from build123d import *

# Parameters (mm, degrees)
BOSS_EXTRUDE1_DEPTH            = 13.97
FILLET1_R                      = 1.27
CBORE_FOR_M8_SHCS1_D           = 9
CBORE_FOR_M8_SHCS1_CBORE_D     = 13.5
CBORE_FOR_M8_SHCS1_CBORE_DEPTH = 4
M4_CLEARANCE_HOLE1_D           = 4.3
SKETCH6_R                      = 4.5
CUT_EXTRUDE1_DEPTH             = 4
BOSS_EXTRUDE3_REACH            = 19.794
SKETCH9_R                      = 6.985
SKETCH9_R_2                    = 2.15


with BuildPart() as part:
    # Sketch1 → Boss-Extrude1 (new body)
    with BuildSketch(Plane.XY):
        with BuildLine():
            Line((-8.897, -5), (-8.897, -21.956))
            ThreePointArc((-8.897, -21.956), (-7.755595126, -24.711595126), (-5, -25.853))
            Line((-5, -25.853), (5, -25.853))
            ThreePointArc((5, -25.853), (7.755595126, -24.711595126), (8.897, -21.956))
            Line((8.897, -21.956), (8.897, -5))
            Line((8.897, -5), (8.897, 5))
            ThreePointArc((8.897, 5), (7.755595126, 7.755595126), (5, 8.897))
            Line((5, 8.897), (-5, 8.897))
            ThreePointArc((-5, 8.897), (-7.755595126, 7.755595126), (-8.897, 5))
            Line((-8.897, 5), (-8.897, -5))
        make_face()
    extrude(amount=BOSS_EXTRUDE1_DEPTH)

    # Fillet1
    fillet1_edges = [part.edges().sort_by_distance(p)[0] for p in [
        (-7.755595126, -24.711595126, 13.97),
        (7.755595126, 7.755595126, 0),
        (8.897, -8.478, 0),
        (7.755595126, -24.711595126, 0),
        (0, -25.853, 0),
        (-7.755595126, -24.711595126, 0),
        (-8.897, -8.478, 0),
        (0, -25.853, 13.97),
        (7.755595126, -24.711595126, 13.97),
        (8.897, -8.478, 13.97),
        (7.755595126, 7.755595126, 13.97),
        (0, 8.897, 13.97),
        (-7.755595126, 7.755595126, 13.97),
        (-8.897, -8.478, 13.97),
        (-7.755595126, 7.755595126, 0),
        (0, 8.897, 0),
    ]]
    fillet(fillet1_edges, radius=FILLET1_R)

    # CBORE for M8 SHCS1 (through all)
    with Locations(Plane.XY.offset(13.97)):
        with Locations((0, 0)):
            CounterBoreHole(CBORE_FOR_M8_SHCS1_D / 2, CBORE_FOR_M8_SHCS1_CBORE_D / 2, CBORE_FOR_M8_SHCS1_CBORE_DEPTH)

    # M4 Clearance Hole1 (through all)
    with Locations(Plane(origin=(8.897, 0, 0), x_dir=(0, 0, -1), z_dir=(1, 0, 0))):
        with Locations((-6.985, -18.233)):
            Hole(M4_CLEARANCE_HOLE1_D / 2)

    # Sketch6 → Cut-Extrude1 (cut)
    with BuildSketch(Plane.XY):
        Circle(SKETCH6_R)
        Polygon((-3.75277675, 6.5), (-7.505553499, 0), (-3.75277675, -6.5), (3.75277675, -6.5), (7.505553499, 0), (3.75277675, 6.5), align=None)
        Polygon((-3.25, 5.629165125), (-6.5, 3.75277675), (-6.5, 0), (-6.5, -3.75277675), (-3.25, -5.629165125), (0, -7.505553499), (3.25, -5.629165125), (6.5, -3.75277675), (6.5, 0), (6.5, 3.75277675), (3.25, 5.629165125), (0, 7.505553499), align=None)
        Polygon((6.5, 3.75277675), (4.758330249, 4.758330249), (6.5, 1.741669751), align=None)
        Polygon((6.5, -3.75277675), (6.5, -1.741669751), (4.758330249, -4.758330249), align=None)
        Polygon((3.75277675, -6.5), (4.758330249, -4.758330249), (3.25, -5.629165125), (1.741669751, -6.5), align=None)
        Polygon((1.741669751, 6.5), (3.25, 5.629165125), (4.758330249, 4.758330249), (3.75277675, 6.5), align=None)
        Polygon((-6.5, 1.741669751), (-4.758330249, 4.758330249), (-6.5, 3.75277675), align=None)
        Polygon((-4.758330249, -4.758330249), (-6.5, -1.741669751), (-6.5, -3.75277675), align=None)
        Polygon((-3.25, -5.629165125), (-4.758330249, -4.758330249), (-3.75277675, -6.5), (-1.741669751, -6.5), align=None)
        Polygon((0, -7.505553499), (1.741669751, -6.5), (-1.741669751, -6.5), align=None)
        Polygon((-3.25, 5.629165125), (-1.741669751, 6.5), (-3.75277675, 6.5), (-4.758330249, 4.758330249), align=None)
        Polygon((7.505553499, 0), (6.5, 1.741669751), (6.5, 0), (6.5, -1.741669751), align=None)
        Polygon((-1.741669751, 6.5), (1.741669751, 6.5), (0, 7.505553499), align=None)
        Polygon((-6.5, 0), (-6.5, 1.741669751), (-7.505553499, 0), (-6.5, -1.741669751), align=None)
    extrude(amount=CUT_EXTRUDE1_DEPTH, mode=Mode.SUBTRACT)

    # Sketch9 → Boss-Extrude3 (add, up to next)
    with BuildSketch(Plane.ZY.offset(8.897), mode=Mode.PRIVATE) as boss_extrude3_sk1:
        with Locations((6.985, -18.233)):
            Circle(SKETCH9_R)
        with Locations((6.985, -18.233)):
            Circle(SKETCH9_R_2, mode=Mode.SUBTRACT)
    boss_extrude3_tool1 = extrude(boss_extrude3_sk1.sketch, amount=-BOSS_EXTRUDE3_REACH, mode=Mode.PRIVATE) - part.part
    add(boss_extrude3_tool1.solids().sort_by_distance((-8.897, -18.233, 0.197566))[0])


solid = part.part
The listing builds one solid part. Answer for the finished solid, in the listing's coordinates (mm). A direction names the side the tool comes from. Round coordinates to 2 decimals unless told otherwise and drop trailing zeros. Order: outer loops, then holes, each group sorted by start corner. A loop starts at its lowest first (then second) coordinate and runs counter-clockwise, first axis right, second up. Notation, with made-up numbers: (-28.75, -3.75) - (25.25, -3.75) arc R24 cw to (25.25, 16.25) - close; hole circle Ø9 at (73, 83.25). An arc over 180 degrees is marked (long way). Write item = value, one per line. Start each with the question number.
1) Section C-C, the plane z = 6 is taken. Write down the section's boundary in (x, y).
2) Given pin 1 (4 mm diameter, centred on x = -1, y = 3, fed in from +Z); pin 2 (7.5 mm diameter, centred on x = 3, y = 0, fed in from -Z); pin 3 (8 mm diameter, centred on x = 0, y = 0, fed in from -Z), each flat-ended and moving along its own axis, determine where each tip first touches the part or whether it passes through.
3) Straight lines are drawn through the part: L1, parallel to Y at x = 0, z = 6.05; L2, parallel to Y at x = 1, z = 8; L3, parallel to Y at x = -3.5, z = 1.25. For each, find the intervals that lie inside material, in ascending order.
4) Section A-A, the plane z = 11.5 is taken. Write down the section's boundary in (x, y).
5) Section B-B, the plane y = -17.5 is taken. Write down the section's boundary in (x, z).
6) For faces 1 (the flat face through (4.4, 1.6, 9.97)), 2 (the cylindrical face through (0.59, 4.46, 6.94)), 3 (the flat face through (-6.5, -3, 2)), 4 (the flat face through (0, -25.853, 7)), 5 (the cylindrical face through (-8.126, -20.948, 13.868)), determine the directions among +Z, -Z, +X, -X, +Y, -Y from which every point of the face is accessible in a straight line to the end or side of a thin tool.
7) Section D-D, the plane y = -2.5 is taken. Write down the section's boundary in (x, z).
8) For a pull along X with two mould halves and no side action, classify faces 6 (the cylindrical face through (8.535, -8.289, 0.382)), 7 (the cylindrical face through (0.07, -25.49, 0.38)), 8 (the flat face through (-3, 6.5, 2)) as released by +X, released by -X, zero draft, split by the parting line, or undercut.
Results list:
q1.outline = (-8.9, -25.15) - (-7.24, -25.15) arc R3.9 ccw to (-5, -25.85) - (5, -25.85) arc R3.9 ccw to (8.9, -21.96) - (8.9, -20.14) - (-8.9, -20.14) - close; (-8.9, -16.32) - (8.9, -16.32) - (8.9, 5) arc R3.9 ccw to (5, 8.9) - (-5, 8.9) arc R3.9 ccw to (-8.9, 5) - close; hole circle Ø9 at (0, 0)
q2.pin_1 = 9.97
q2.pin_2 = 4
q2.pin_3 = through
q3.L1 = -25.85 to -20.17, -16.3 to -4.5, 4.5 to 8.9
q3.L2 = -25.85 to -20.13, -16.34 to -4.39, 4.39 to 8.9
q3.L3 = -25.85 to -6.5, 6.5 to 8.9
q4.outline = (-8.9, -23.56) - (-8.55, -23.56) arc R3.9 ccw to (-5, -25.85) - (5, -25.85) arc R3.9 ccw to (8.9, -21.96) - (8.9, 5) arc R3.9 ccw to (5, 8.9) - (-5, 8.9) arc R3.9 ccw to (-8.9, 5) - close; hole circle Ø13.5 at (0, 0)
q5.outline = (-8.9, 0.04) - (-7.94, 0.04) arc R1.27 ccw to (-7.63, 0) - (7.63, 0) arc R1.27 ccw to (8.9, 1.27) - (8.9, 4.96) - (-8.9, 4.96) - close; (-8.9, 9.01) - (8.9, 9.01) - (8.9, 12.7) arc R1.27 ccw to (7.63, 13.97) - (-7.63, 13.97) arc R1.27 ccw to (-7.94, 13.93) - (-8.9, 13.93) - close
q6.face_1 = +Z
q6.face_2 = +Z, -Z
q6.face_3 = -Z
q6.face_4 = +Z, -Z, +X, -X, -Y
q6.face_5 = +Z, -X, -Y
q7.outline = (-8.9, 1.27) arc R1.27 ccw to (-7.63, 0) - (-6.5, 0) - (-6.5, 4) - (-3.74, 4) - (-3.74, 9.97) - (-6.27, 9.97) - (-6.27, 13.97) - (-7.63, 13.97) arc R1.27 ccw to (-8.9, 12.7) - close; (3.74, 4) - (6.5, 4) - (6.5, 0) - (7.63, 0) arc R1.27 ccw to (8.9, 1.27) - (8.9, 12.7) arc R1.27 ccw to (7.63, 13.97) - (6.27, 13.97) - (6.27, 9.97) - (3.74, 9.97) - close
q8.face_6 = released by +X
q8.face_7 = zero draft
q8.face_8 = undercut
